Job drawing, mm, ordinate dimensions from the low corner. One solid piece. A direction names the side the tool comes from. Round coordinates to 2 decimals unless told otherwise and drop trailing zeros. Order: outer loops, then holes, each group sorted by start corner. A loop starts at its lowest first (then second) coordinate and runs counter-clockwise, first axis right, second up. Notation, with made-up numbers: (10, 32.5) -> (30, 32.5) arc R31 cw to (30, 59.5) -> close; hole circle Ø8 at (-8, 89.5). An arc over 180 degrees is marked (long way). Answer as a JSON object with one key per item and string values. Group by question number.
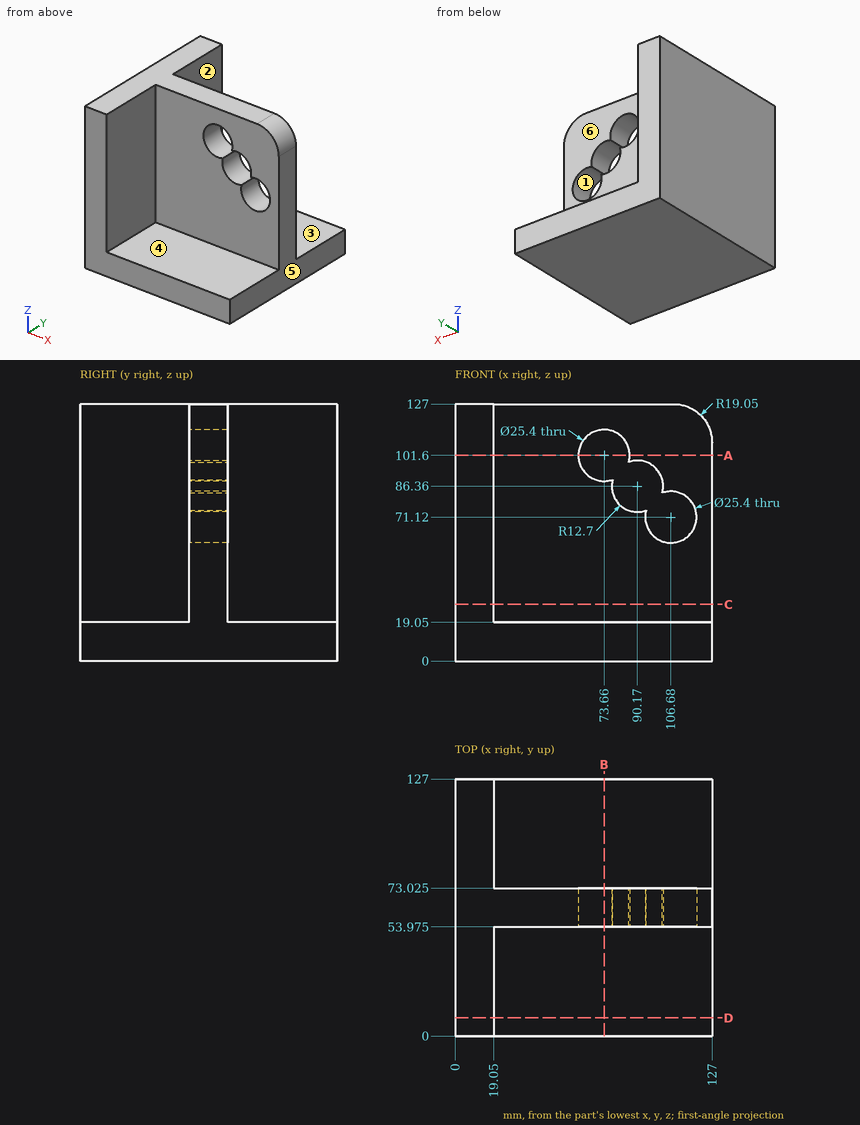
Q1. Wall check: line 1 (Z direction, x = 106, y = 65); line 2 (X direction, y = 68, z = 101); line 3 (X direction, y = 58.25, z = 101.6). Give the ranges that are in metal, low to high. Write a range as [from, to].
Q2. Band-saw the part on A-A (z = 101.6). List the corners of the cut face in (x, y) (3 decimals).
Q3. Band-saw the part on B-B (x = 73.66). List the corners of the cut face in (y, z) (3 decimals).
Q4. Band-saw the part on C-C (z = 28). List the corners of the cut face in (x, y) (3 decimals), plus the area to 3 significant figures.
Q5. Which spindle directions (+Z, -Z, +X, -X, +Y, -Y) get a long thin tool onto all of the face, cutting with end or side? Do the marked faces 4, 5 and 6. Say none if no direction does.
Q6. Drop flat-ended pins along their axis: pin 1 Ø2 at (x, y) = (104, 22.5) entering from +Z; pin 2 Ø2 at (y, z) = (78, 110) entering from +X. Give the stop position or say it passes through.
Q7. Two-plate mould, pull along Z, no slides. Class the marked faces 1, 2 and 3: +Z half, -Z half, draft (parallel to the pull), parting line (faces both ways), or undercut.
Q8. Band-saw the part on D-D (y = 9). List the corners of the cut face in (x, z), plus the area to 3 significant figures.
Completed:
{
 "1": {"line 1": "[0, 58.44], [83.8, 127]", "line 2": "[0, 60.97], [86.35, 127]", "line 3": "[0, 60.96], [86.36, 127]"},
 "2": {"outline": "(0, 0) -> (19.05, 0) -> (19.05, 53.975) -> (60.96, 53.975) -> (60.96, 73.025) -> (19.05, 73.025) -> (19.05, 127) -> (0, 127) -> close; (86.36, 53.975) -> (127, 53.975) -> (127, 73.025) -> (86.36, 73.025) -> close"},
 "3": {"outline": "(0, 0) -> (127, 0) -> (127, 19.05) -> (73.025, 19.05) -> (73.025, 88.9) -> (53.975, 88.9) -> (53.975, 19.05) -> (0, 19.05) -> close; (53.975, 114.3) -> (73.025, 114.3) -> (73.025, 127) -> (53.975, 127) -> close"},
 "4": {"outline": "(0, 0) -> (19.05, 0) -> (19.05, 53.975) -> (127, 53.975) -> (127, 73.025) -> (19.05, 73.025) -> (19.05, 127) -> (0, 127) -> close", "area": "4,480 mm2"},
 "5": {"face 4": "+Z, +X, -Y", "face 5": "+Z, -Z, +X, +Y, -Y", "face 6": "+Z, +X, +Y"},
 "6": {"pin 1": "z = 19.05", "pin 2": "x = 19.05"},
 "7": {"face 1": "undercut", "face 2": "draft", "face 3": "+Z half"},
 "8": {"outline": "(0, 0) -> (127, 0) -> (127, 19.05) -> (19.05, 19.05) -> (19.05, 127) -> (0, 127) -> close", "area": "4,480 mm2"}
}
